For this review, take the finished solid that the model builds, in its own axes (mm). A direction names the side the tool comes from. Give positions to 0.01 mm unless a question says otherwise; leave off trailing zeros. Order: outer loops, then holes, each group sorted by start corner. A loop starts at its lowest first (then second) coordinate and runs counter-clockwise, first axis right, second up.
Item 1: The part is to be moulded in two halves that separate along Y. For faces 6 (the cylindrical face through (-28.547, 1.256, 21.825)), 7 (the flat face through (20.422, 0, 41)), 8 (the cylindrical face through (22.95, 0.35, 52.38)), 9 (the flat face through (-27, 0, 31.75)), say which applies: released by +Y, released by -Y, zero draft, split by the parting line, or undercut.
Item 2: For P1, Ø5, axis at y = 1, z = 42, coming from the +X side; P2, Ø1, axis at x = 26.5, y = 2, coming from the +Z side; P3, Ø12, axis at y = -10, z = 27, coming from the +X side, all flat-tipped, find the tip position at first contact; note any pin that passes through.
Item 3: For probe 1 along Y at (x, z) = (0, 10.25) (1 decimal); probe 2 along X at (y, z) = (7.5, 33); probe 3 along Z at (x, y) = (8, -21.5), list the stretches that pass through material, from the lowest coordinate up.
Item 4: Consider section D-D (x = 0). Give the boundary of the cut face in (y, z) (1 decimal), plus the area to 3 significant figures.
Item 5: Consider section A-A (z = 35.5). Give the boundary of the cut face in (x, y) (3 decimals), plus the area to 3 significant figures.
Item 6: Consider section B-B (z = 44.45). Give the number of separate pieces and of enclosed holes in the cut face, plus the area to 3 significant figures.
Item 7: Machinability: for faces 1 (the cylindrical face through (-22.88, -0.35, 52.38)), 2 (the flat face through (8.3, 0.4, 12.573)), 3 (the flat face through (25.4, -6, 50)), 4 (the flat face through (-25.4, -6, 39)), 5 (the flat face through (-18, 0, 57.15)), which of the approach directions +Z, -Z, +X, -X, +Y, -Y give a long, thin tool a straight path to every point of the face, cutting with its end or side? Answer none if there is none.
```python
from build123d import *

# Parameters (mm, degrees)
SKETCH1_R                = 28.575
OD_DON_T_CARE_DEPTH      = 57.15
SKETCH3_W                = 25.4
SKETCH3_H                = 44.577
SLOT_DEPTH               = 50.8
SKETCH4_R                = 7.9375
F_5_8_THROUGH_HOLE_DEPTH = 61.167850045
SKETCH5_OUTSIDE_W        = 78.948
SKETCH5_OUTSIDE_H        = 78.948
SKETCH5_OUTSIDE_W_2      = 53.975
SKETCH5_OUTSIDE_H_2      = 51.195336702
FLAT_SURFACE_DEPTH       = 25.4
SKETCH2_R                = 3.175
F_1_4_THROUGH_HOLE_DEPTH = 84.641818189
SKETCH6_R                = 7.9375
CUT_EXTRUDE1_DEPTH       = 4.9784
CUT_EXTRUDE2_DEPTH       = 70.994169563
CUT_EXTRUDE2_DEPTH_BACK  = 25.4
CUT_EXTRUDE3_START       = -4.9784
SKETCH8_R                = 7.9375
CUT_EXTRUDE3_DEPTH       = 4.9784


with BuildPart() as part:
    # Sketch1 → OD Don't Care (new body)
    with BuildSketch(Plane.XY):
        Circle(SKETCH1_R)
    extrude(amount=OD_DON_T_CARE_DEPTH)

    # Sketch3 → Slot (cut, symmetric)
    with BuildSketch(Plane(origin=(0, 0, 0), x_dir=(1, 0, 0), z_dir=(0, 1, 0))):
        with Locations((0, -34.8615)):
            Rectangle(SKETCH3_W, SKETCH3_H)
    extrude(amount=SLOT_DEPTH, both=True, mode=Mode.SUBTRACT)

    # Sketch4 → 5/8" Through Hole (cut, through all)
    with BuildSketch(Plane.XY.offset(12.573)):
        Circle(SKETCH4_R)
    extrude(amount=-F_5_8_THROUGH_HOLE_DEPTH, mode=Mode.SUBTRACT)

    # Sketch5 outside → Flat Surface (cut)
    with BuildSketch(Plane.XY.offset(57.15)):
        Rectangle(SKETCH5_OUTSIDE_W, SKETCH5_OUTSIDE_H)
        with Locations((-1.5875, 0)):
            Rectangle(SKETCH5_OUTSIDE_W_2, SKETCH5_OUTSIDE_H_2, mode=Mode.SUBTRACT)
    extrude(amount=-FLAT_SURFACE_DEPTH, mode=Mode.SUBTRACT)

    # Sketch2 → 1/4" Through Hole (cut, through all)
    with BuildSketch(Plane(origin=(25.4, 0, 0), x_dir=(0, 0, -1), z_dir=(1, 0, 0))):
        with Locations((-44.45, 0)):
            Circle(SKETCH2_R)
    extrude(amount=-F_1_4_THROUGH_HOLE_DEPTH, mode=Mode.SUBTRACT)

    # Sketch6 → Cut-Extrude1 (cut)
    with BuildSketch(Plane(origin=(25.4, 0, 0), x_dir=(0, 0, -1), z_dir=(1, 0, 0))):
        with Locations((-44.45, 0)):
            Circle(SKETCH6_R)
    extrude(amount=-CUT_EXTRUDE1_DEPTH, mode=Mode.SUBTRACT)

    # Sketch7 → Cut-Extrude2 (cut, two sides: drawn at the far end of the back side and taken through both)
    with BuildSketch(Plane.XY.offset(57.15).offset(-CUT_EXTRUDE2_DEPTH_BACK)):
        Polygon((-25.4, -159.463065209), (-25.4, -13.090860361), (-25.4, 13.090860361), (-25.4, 159.463065209), (-318.144409696, 159.463065209), (-318.144409696, -159.463065209), align=None)
    extrude(amount=CUT_EXTRUDE2_DEPTH + CUT_EXTRUDE2_DEPTH_BACK, mode=Mode.SUBTRACT)

    # Sketch8 → Cut-Extrude3 (cut)
    with BuildSketch(Plane.ZY.offset(25.4).offset(CUT_EXTRUDE3_START)):
        with Locations(Location((44.45, 0, 0), (0, 0, 180))):
            Circle(SKETCH8_R)
    extrude(amount=CUT_EXTRUDE3_DEPTH, mode=Mode.SUBTRACT)


solid = part.part
```
Resolved:
1. face 6: split by the parting line
1. face 7: undercut
1. face 8: undercut
1. face 9: zero draft
2. P1: stops at x = 20.42
2. P2: stops at z = 31.75
2. P3: stops at x = 28.29
3. probe 1: y = -28.6 to -7.9, 7.9 to 28.6
3. probe 2: x = -25.4 to -12.7, 12.7 to 25.4
3. probe 3: z = 0 to 12.57
4. outline: (-28.6, 0) - (-7.9, 0) - (-7.9, 12.6) - (-28.6, 12.6) - close; (7.9, 0) - (28.6, 0) - (28.6, 12.6) - (7.9, 12.6) - close
4. area: 519 mm2
5. outline: (-25.4, -13.091) arc R28.575 ccw to (-12.7, -25.598) - (-12.7, 25.598) arc R28.575 ccw to (-25.4, 13.091) - close; (12.7, -25.598) arc R28.575 ccw to (25.4, -13.091) - (25.4, 13.091) arc R28.575 ccw to (12.7, 25.598) - close
5. area: 1,050 mm2
6. separate pieces: 4
6. enclosed holes: 0
6. area: 795 mm2
7. face 1: -X
7. face 2: +Z, +Y, -Y
7. face 3: +Z, +X, +Y, -Y
7. face 4: +Z, -X, +Y, -Y
7. face 5: +Z, +X, -X, +Y, -Y
